The figure shows three views and two pictorial views of one solid part (mm, origin at its lowest corner). Answer the questions. A direction names the side the tool comes from. Give positions to 0.01 mm unless a question says otherwise; leave off trailing zeros. Order: outer loops, then holes, each group sorted by start corner. A loop starts at its lowest first (then second) coordinate and runs counter-clockwise, first axis right, second up. Notation, with made-up numbers: (30, 36) - (82, 36) arc R28 ccw to (82, 70) - close; hole circle Ø3 at (4.25, -21). An arc over 180 degrees is marked (long way). Use a Markdown table: item, result. Add a question column.
1. A cutting plane is placed at D-D on x = 15.25. Determine the outline of the cut face in (y, z).
2. A cutting plane is placed at A-A on z = 8.5. State how many separate pieces and enclosed holes the cut face has, and give its area (3 significant figures).
3. Flat-ended cylindrical pins translate along their axes: P1, Ø1.5, axis at y = 8, z = 3, coming from the +X side; P2, Ø3, axis at x = 9.525, y = 6.35, coming from the +Z side. Find the tip coordinate at first contact, or state that the pin passes through.
4. Consider L1, parallel to Y at x = 9.5, z = 7.5; L2, parallel to X at y = 20, z = 11.25; L3, parallel to Y at x = 8, z = 8. Determine where each line is inside the solid, lowest interval first.
5. For a pull along X with two mould halves and no side action, classify the marked faces 1, 2 and 3 as released by +X, released by -X, zero draft, split by the parting line, or undercut.
6. Which of the six approach directions +Z, -Z, +X, -X, +Y, -Y give full straight-line access (tool end or side, diameter ignored) to the marked faces 4 and 5?
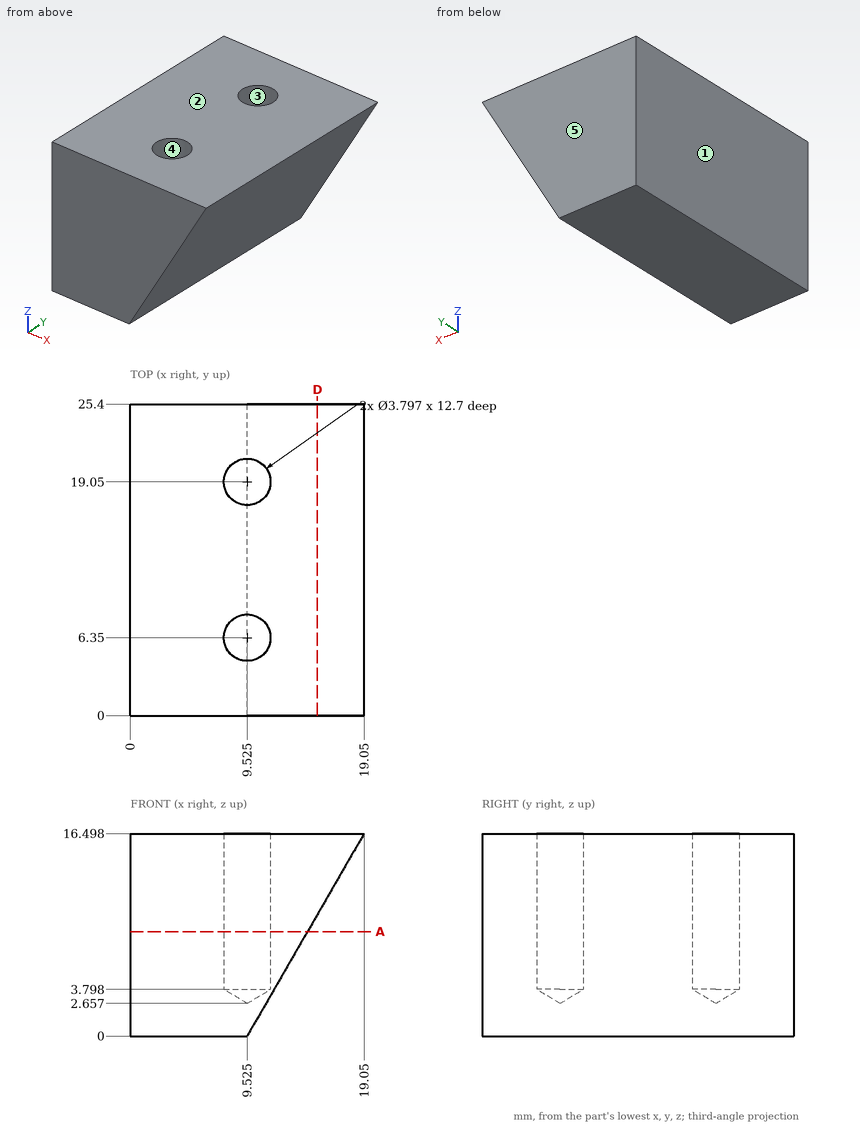
Output values:
| question | item | result |
|---|---|---|
| 1 | outline | (0, 9.92) - (25.4, 9.92) - (25.4, 16.5) - (0, 16.5) - close |
| 2 | separate pieces | 1 |
| 2 | enclosed holes | 2 |
| 2 | area | 344 mm² |
| 3 | P1 | x = 11.69 |
| 3 | P2 | z = 3.56 |
| 4 | L1 | 0 to 4.45, 8.25 to 17.15, 20.95 to 25.4 |
| 4 | L2 | 0 to 7.88, 11.17 to 16.02 |
| 4 | L3 | 0 to 5.22, 7.48 to 17.92, 20.18 to 25.4 |
| 5 | face 1 | released by -X |
| 5 | face 2 | zero draft |
| 5 | face 3 | undercut |
| 6 | face 4 | +Z |
| 6 | face 5 | +Z, -Z, +X, -X, +Y |
